```python
from build123d import *

# Parameters (mm, degrees)
ESTRUSIONE_ESTRUSIONE1_DEPTH = 10.9


with BuildPart() as part:
    # Schizzo1 → Estrusione-Estrusione1 (new body)
    with BuildSketch(Plane(origin=(0, 0, 0), x_dir=(1, 0, 0), z_dir=(0, 1, 0))):
        with BuildLine():
            ThreePointArc((-2.151851846, -3.489918858), (-2.814062516, 2.981786738), (3.608517792, 1.946432465))
            ThreePointArc((3.608517792, 1.946432465), (4.39902179, 4.588421002), (7.041010327, 3.797917005))
            ThreePointArc((7.041010327, 3.797917005), (-5.49085365, 5.818120504), (-4.198735404, -6.809597712))
            ThreePointArc((-4.198735404, -6.809597712), (-4.835133005, -4.126316535), (-2.151851846, -3.489918858))
        make_face()
        with BuildLine():
            ThreePointArc((-1.225293577, -5.149758315), (-1.47261754, -4.199287741), (-2.151851846, -3.489918858))
            ThreePointArc((-2.151851846, -3.489918858), (-4.835133005, -4.126316535), (-4.198735404, -6.809597712))
            ThreePointArc((-4.198735404, -6.809597712), (-2.224823052, -6.852434379), (-1.225293577, -5.149758315))
        make_face()
        with BuildLine():
            ThreePointArc((7.041010327, 3.797917005), (4.39902179, 4.588421002), (3.608517792, 1.946432465))
            ThreePointArc((3.608517792, 1.946432465), (5.802163148, 0.981516091), (7.27476406, 2.872174735))
            ThreePointArc((7.27476406, 2.872174735), (7.215422704, 3.349573823), (7.041010327, 3.797917005))
        make_face()
    extrude(amount=ESTRUSIONE_ESTRUSIONE1_DEPTH)


solid = part.part
```
Work out the finished part from the listing and answer in its coordinate system (mm). Round coordinates to 2 decimals unless told otherwise and drop trailing zeros. Loops run counter-clockwise (first coordinate to the right, second up) from the corner with the lowest first, then second, coordinate; pieces in that order, holes last.
(1) The part is cut by section B-B, the plane x = 0. Give the vertices of the cut face in (y, z).
Computed values:
outline: (0, -8) - (10.9, -8) - (10.9, -4.1) - (0, -4.1) - close
(2) The part is cut by section C-C, the plane z = 0. Give the vertices of the cut face in (x, y).
Computed values:
outline: (-8, 0) - (-4.1, 0) - (-4.1, 10.9) - (-8, 10.9) - close
(3) Find the intervals of material crossed by L1, parallel to Z at x = 0, y = 3; L2, parallel to Z at x = -2.75, y = 6.25, in increasing order.
Computed values:
L1: z = -8 to -4.1
L2: z = -7.51 to -3.04, 3.04 to 7.05
(4) The mould has two halves that part along Z. Classify faces 1 (the cylindrical face through (-2.9, 5.4, -2.9)), 2 (the flat face through (-2, 0, -4)), 3 (the cylindrical face through (-5.34, 5.374, -5.957)): pulls with the +Z half, pulls with the -Z half, needs draft (parallel to the pull), parting line crosses it, or undercut.
Computed values:
face 1: undercut
face 2: needs draft
face 3: parting line crosses it
(5) The part is cut by section D-D, the plane y = 10. Give the vertices of the cut face in (x, z), and give its area (3 significant figures).
Computed values:
outline: (-4.2, 6.81) arc R8 ccw (long way) to (7.04, -3.8) arc R1.95 ccw to (3.61, -1.95) arc R4.1 cw (long way) to (-2.15, 3.49) arc R1.95 ccw to start
area: 98.4 mm2
(6) The part is cut by section A-A, the plane z = -2.25. Give the vertices of the cut face in (x, y).
Computed values:
outline: (-7.68, 0) - (-3.43, 0) - (-3.43, 10.9) - (-7.68, 10.9) - close; (3.43, 0) - (7.17, 0) - (7.17, 10.9) - (3.43, 10.9) - close
(7) Each of these flat-tipped pins is pushed along its axis until it touches: P1, Ø8, axis at x = -2.5, z = -1, coming from the +Y side; P2, Ø3, axis at x = 4, y = 5, coming from the +Z side; P3, Ø3, axis at y = 8.5, z = -4.5, coming from the -X side. Where does it stop, or does it pass through?
Computed values:
P1: stops at y = 10.9
P2: stops at z = -0.92
P3: stops at x = -7.42
